Design review of the part built by this model. Coordinates are the model's own, in mm. Coordinates: 2 decimals unless noted, no trailing zeros. Write each loop counter-clockwise with the first axis right and the second up, starting at its lowest first coordinate (ties: lowest second). Pieces come first, ordered by that corner, then holes. Notation, with made-up numbers: (17.25, 80) - (22.25, 80) arc R8 ccw to (22.25, 93) - close; hole circle Ø6 at (45.5, 55). An arc over 180 degrees is marked (long way). Answer as a JSON object with one key per item and string values.
```python
from build123d import *

# Parameters (mm, degrees)
F1_DEPTH = 1
F2_SIZE  = 0.5
F3_R     = 2
F4_DEPTH = 25


with BuildPart() as f1:
    # F0 (on Top) → F1 (new body)
    with BuildSketch(Plane.XY):
        Polygon((-7, -2.5), (-7, -7), (-2.5, -7), (-2.5, -4.5), (2.5, -4.5), (2.5, -7), (7, -7), (7, -2.5), (4.5, -2.5), (4.5, 2.5), (7, 2.5), (7, 7), (2.5, 7), (2.5, 4.5), (-2.5, 4.5), (-2.5, 7), (-7, 7), (-7, 2.5), (-4.5, 2.5), (-4.5, -2.5), align=None)
    extrude(amount=F1_DEPTH)

    # F2
    f2_edges = [f1.edges().sort_by_distance(p)[0] for p in [
        (-7, -7, 0.5),
        (-2.5, -7, 0.5),
        (-7, -2.5, 0.5),
        (-7, 2.5, 0.5),
        (-7, 7, 0.5),
        (-2.5, 7, 0.5),
        (2.5, 7, 0.5),
        (7, 7, 0.5),
        (7, -2.5, 0.5),
        (7, -7, 0.5),
        (2.5, -7, 0.5),
        (7, 2.5, 0.5),
    ]]
    chamfer(f2_edges, length=F2_SIZE)

    # F3 (on face) → F4 (cut)
    with BuildSketch(Plane.XY.offset(1)):
        Circle(F3_R)
    extrude(amount=-F4_DEPTH, mode=Mode.SUBTRACT)


solid = f1.part
```
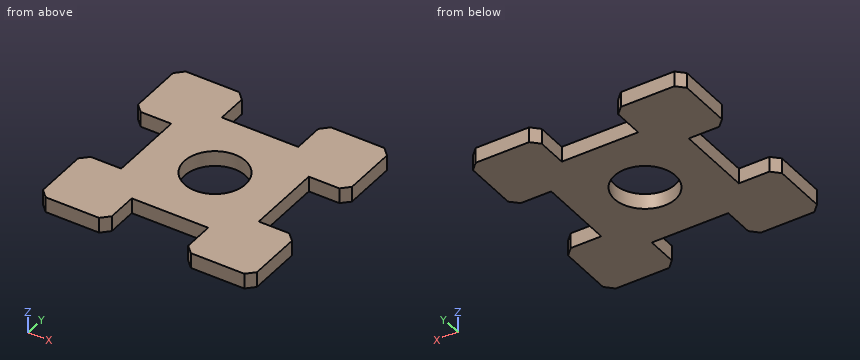
(1) Take a section at A-A, the plane x = -5.5. Write out the cut boundary in (y, z), and give its area (3 significant figures).
Solved:
{"outline": "(-7, 0) - (-2.5, 0) - (-2.5, 1) - (-7, 1) - close; (2.5, 0) - (7, 0) - (7, 1) - (2.5, 1) - close", "area": "9.00 mm^2"}
(2) To check wall thickness, follow line 1 (Y direction, x = 0, z = 0.65); line 2 (X direction, y = 5, z = 0.75); line 3 (Y direction, x = -2.25, z = 0.85). State the ranges of each line that lie inside material, in increasing order. Write a range as from..to.
Solved:
{"line 1": "y = -4.5..-2, 2..4.5", "line 2": "x = -7..-2.5, 2.5..7", "line 3": "y = -4.5..4.5"}
